Verification items for the finished model (mm, model axes). A direction names the side the tool comes from. Round coordinates to 2 decimals unless told otherwise and drop trailing zeros. Order: outer loops, then holes, each group sorted by start corner. A loop starts at its lowest first (then second) coordinate and runs counter-clockwise, first axis right, second up. Notation, with made-up numbers: (-38.75, 24.5) -> (-24.75, 24.5) arc R22 ccw to (-24.75, 58.5) -> close; hole circle Ø2 at (43, 0). An arc over 180 degrees is marked (long way). Put each result on its own line as item: value.
from build123d import *

# Parameters (mm, degrees)
SKETCH_W        = 56
SKETCH_H        = 56
PAD_DEPTH       = 5
SKETCH001_R     = 10
PAD001_DEPTH    = 7.5
SKETCH002_R     = 3.15
POCKET_DEPTH    = 12.501
SKETCH003_R     = 5
PAD002_DEPTH    = 23
SKETCH004_R     = 1.6
POCKET001_DEPTH = 7.5
SKETCH006_R     = 1.6
POCKET002_DEPTH = 7.5
SKETCH007_R     = 1.6
POCKET003_DEPTH = 7.5
SKETCH008_R     = 1.6
POCKET004_DEPTH = 7.5


with BuildPart() as part:
    # Sketch → Pad (new body)
    with BuildSketch(Plane.XY):
        Rectangle(SKETCH_W, SKETCH_H)
    extrude(amount=PAD_DEPTH)

    # Sketch001 (on Face5 of Pad) → Pad001 (join)
    with BuildSketch(Plane(origin=(0, 0, 0), x_dir=(1, 0, 0), z_dir=(0, 0, -1))):
        Circle(SKETCH001_R)
    extrude(amount=PAD001_DEPTH)

    # Sketch002 (on Face8 of Pad001) → Pocket (cut, through all)
    with BuildSketch(Plane(origin=(0, 0, -7.5), x_dir=(1, 0, 0), z_dir=(0, 0, -1))):
        Circle(SKETCH002_R)
    extrude(amount=-POCKET_DEPTH, mode=Mode.SUBTRACT)

    # Sketch003 (on Face4 of Pocket) → Pad002 (join)
    with BuildSketch(Plane(origin=(0, 0, 0), x_dir=(1, 0, 0), z_dir=(0, 0, -1))):
        with Locations((-21.5, 21.5)):
            Circle(SKETCH003_R)
        with Locations((21.5, 21.5)):
            Circle(SKETCH003_R)
        with Locations((-21.5, -21.5)):
            Circle(SKETCH003_R)
        with Locations((21.5, -21.5)):
            Circle(SKETCH003_R)
    extrude(amount=PAD002_DEPTH)

    # Sketch004 (on Face15 of Pad002) → Pocket001 (cut)
    with BuildSketch(Plane(origin=(0, 0, -23), x_dir=(1, 0, 0), z_dir=(0, 0, -1))):
        with Locations((-21.5, 21.5)):
            Circle(SKETCH004_R)
    extrude(amount=-POCKET001_DEPTH, mode=Mode.SUBTRACT)

    # Sketch006 (on Face14 of Pocket001) → Pocket002 (cut)
    with BuildSketch(Plane(origin=(0, 0, -23), x_dir=(1, 0, 0), z_dir=(0, 0, -1))):
        with Locations((21.5, 21.5)):
            Circle(SKETCH006_R)
    extrude(amount=-POCKET002_DEPTH, mode=Mode.SUBTRACT)

    # Sketch007 (on Face15 of Pocket002) → Pocket003 (cut)
    with BuildSketch(Plane(origin=(0, 0, -23), x_dir=(1, 0, 0), z_dir=(0, 0, -1))):
        with Locations((-21.5, -21.5)):
            Circle(SKETCH007_R)
    extrude(amount=-POCKET003_DEPTH, mode=Mode.SUBTRACT)

    # Sketch008 (on Face17 of Pocket003) → Pocket004 (cut)
    with BuildSketch(Plane(origin=(0, 0, -23), x_dir=(1, 0, 0), z_dir=(0, 0, -1))):
        with Locations((21.5, -21.5)):
            Circle(SKETCH008_R)
    extrude(amount=-POCKET004_DEPTH, mode=Mode.SUBTRACT)


solid = part.part
Item 1: Section check A-A on x = 0. Record the boundary of the cut face in (y, z).
Check sheet entries:
outline: (-28, 0) -> (-10, 0) -> (-10, -7.5) -> (-3.15, -7.5) -> (-3.15, 5) -> (-28, 5) -> close; (3.15, -7.5) -> (10, -7.5) -> (10, 0) -> (28, 0) -> (28, 5) -> (3.15, 5) -> close
Item 2: Section check B-B on z = -20. Record the boundary of the cut face in (x, y).
Check sheet entries:
outline: circle Ø10 at (-21.5, -21.5); circle Ø10 at (-21.5, 21.5); circle Ø10 at (21.5, -21.5); circle Ø10 at (21.5, 21.5); hole circle Ø3.2 at (-21.5, -21.5); hole circle Ø3.2 at (-21.5, 21.5); hole circle Ø3.2 at (21.5, -21.5); hole circle Ø3.2 at (21.5, 21.5)
Item 3: Gauge pin test, flat ends, axial feed: pin 1 Ø6 at (x, y) = (3, -1) entering from -Z; pin 2 Ø4 at (y, z) = (-19.5, -16.5) entering from -X; pin 3 Ø1 at (x, y) = (-21, 21) entering from -Z. Record the tip position at first contact, or that the pin passes through.
Check sheet entries:
pin 1: stops at z = -7.5
pin 2: stops at x = -26.5
pin 3: stops at z = -15.5
Item 4: Tool access check on faces 1 (the cylindrical face through (-2.17, 9.76, -3.7)), 2 (the flat face through (-2.4, -2.4, -7.5)). Record the directions out of +Z, -Z, +X, -X, +Y, -Y that give a thin tool (end or side, any length) a straight path to the whole face; none if there is none.
Check sheet entries:
face 1: -Z
face 2: -Z, +X, -X, +Y, -Y
Item 5: Material ranges on L1, parallel to Y at x = -21.5, z = -17.5; L2, parallel to X at y = 0, z = -2.5, recorded low to high. Write a range as [from, to].
Check sheet entries:
L1: y = [-26.5, -23.1], [-19.9, -16.5], [16.5, 19.9], [23.1, 26.5]
L2: x = [-10, -3.15], [3.15, 10]
Item 6: Section check D-D on z = -6.75. Record the boundary of the cut face in (x, y).
Check sheet entries:
outline: circle Ø10 at (-21.5, -21.5); circle Ø10 at (-21.5, 21.5); circle Ø20 at (0, 0); circle Ø10 at (21.5, -21.5); circle Ø10 at (21.5, 21.5); hole circle Ø6.3 at (0, 0)
Item 7: Release check for a two-part mould opening along X. For faces 3 (the flat face through (28, 0, 2)), 4 (the cylindrical face through (-22.58, 26.38, -11.34)), 5 (the flat face through (-23, -23, -23)) record: +X half, -X half, draft (parallel to the pull), parting line (faces both ways), or undercut.
Check sheet entries:
face 3: +X half
face 4: undercut
face 5: draft
